For this review, take the finished solid that the model builds, in its own axes (mm). A direction names the side the tool comes from. Give positions to 0.01 mm unless a question says otherwise; leave off trailing zeros. Write each loop counter-clockwise with the first axis right and the second up, starting at its lowest first coordinate (ties: lowest second). Pieces come first, ordered by that corner, then holes. Notation, with made-up numbers: M 5.5,25 L 39.5,25 A22 ccw 39.5,39 Z; hole C 63.5,72.5 d6. An arc over 180 degrees is marked long. One line per item, written item: value. Start each with the question number.
Item 1: Clearance check with flat-ended pins moving along their axes: pin 1 Ø6 at (x, z) = (-14, -16.5) entering from +Y; pin 2 Ø6 at (y, z) = (24, -9) entering from +X; pin 3 Ø8 at (y, z) = (10, -28) entering from +X. State where each tip first meets the part, or that it passes through.
Item 2: Consider section B-B, the plane z = -27.5. Write out the cut boundary in (x, y).
Item 3: Consider section A-A, the plane x = -13. Write out the cut boundary in (y, z), and give its area (3 significant figures).
Item 4: Tool access review of faces 5 (the face through (-36, 27, -20)), 6 (the face through (-38, 40, -20)): name each direction out of +Z, -Z, +X, -X, +Y, -Y from which nothing blocks a thin tool from reaching the whole face with its end or side.
Item 5: Consider section D-D, the plane z = -20.5. Write out the cut boundary in (x, y).
Item 6: Consider section C-C, the plane y = 27. Write out the cut boundary in (x, z).
Item 7: Mouldability with a two-part tool opening along Z and no side actions: class faces 1 (the face through (-37.972, 24.804, -12.012)), 2 (the face through (-32, 8, -40)), 3 (the face through (0, 2, -20)), 4 (the face through (-13.488, 2.028, -25.304)) as released by +Z, released by -Z, zero draft, split by the parting line, or undercut.
Item 8: To check wall thickness, follow probe 1 along Z at (x, y) = (-13, 2.2); probe 2 along Y at (x, z) = (-38.35, -12.5); probe 3 along X at (y, z) = (30, -7). State the ranges of each line that lie inside material, in increasing order.
```python
from build123d import *

# Parameters (mm, degrees)
SCHIZZO1_W                   = 40
SCHIZZO1_H                   = 40
ESTRUSIONE_ESTRUSIONE1_DEPTH = 4
SCHIZZO2_W                   = 4
SCHIZZO2_H                   = 40
ESTRUSIONE_ESTRUSIONE2_DEPTH = 36
SMUSSO1_SIZE                 = 10
FORO_PER_VITE_M4_1_D         = 4.5
FORO_PER_VITE_M4_1_DEPTH     = 9
FORO_PER_VITE_M4_1_TIP       = 1.351936393
FORO_PER_VITE_M4_3_D         = 4.5
FORO_PER_VITE_M4_3_DEPTH     = 9
FORO_PER_VITE_M4_3_TIP       = 1.351936393


with BuildPart() as part:
    # Schizzo1 → Estrusione-Estrusione1 (new body)
    with BuildSketch(Plane(origin=(0, 0, 0), x_dir=(1, 0, 0), z_dir=(0, 1, 0))):
        with Locations((-20, 20)):
            Rectangle(SCHIZZO1_W, SCHIZZO1_H)
    extrude(amount=ESTRUSIONE_ESTRUSIONE1_DEPTH)

    # Schizzo2 → Estrusione-Estrusione2 (add)
    with BuildSketch(Plane(origin=(0, 4, 0), x_dir=(1, 0, 0), z_dir=(0, 1, 0))):
        with Locations((-38, 20)):
            Rectangle(SCHIZZO2_W, SCHIZZO2_H)
    extrude(amount=ESTRUSIONE_ESTRUSIONE2_DEPTH)

    # Smusso1
    smusso1_edges = [part.edges().sort_by_distance(p)[0] for p in [
        (-36, 4, -20),
    ]]
    chamfer(smusso1_edges, length=SMUSSO1_SIZE)

    # Foro per Vite M4-1
    with Locations(Plane(origin=(0, 0, 0), x_dir=(-1, 0, 0), z_dir=(0, -1, 0))):
        with Locations((13, 27.5), (13, 12.5)):
            Hole(FORO_PER_VITE_M4_1_D / 2, depth=FORO_PER_VITE_M4_1_DEPTH)
            with Locations((0, 0, -(FORO_PER_VITE_M4_1_DEPTH + FORO_PER_VITE_M4_1_TIP / 2))):  # 118° drill point
                Cone(0, FORO_PER_VITE_M4_1_D / 2, FORO_PER_VITE_M4_1_TIP, mode=Mode.SUBTRACT)

    # Foro per Vite M4-3
    with Locations(Plane.ZY.offset(40)):
        with Locations((-27.5, 27), (-12.5, 27)):
            Hole(FORO_PER_VITE_M4_3_D / 2, depth=FORO_PER_VITE_M4_3_DEPTH)
            with Locations((0, 0, -(FORO_PER_VITE_M4_3_DEPTH + FORO_PER_VITE_M4_3_TIP / 2))):  # 118° drill point
                Cone(0, FORO_PER_VITE_M4_3_D / 2, FORO_PER_VITE_M4_3_TIP, mode=Mode.SUBTRACT)


solid = part.part
```
Model answer:
1. pin 1: stops at y = 4
1. pin 2: stops at x = -36
1. pin 3: stops at x = -28
2. outline: M -40,0 L -15.25,0 L -15.25,4 L -26,4 L -36,14 L -36,24.75 L -40,24.75 Z; M -40,29.25 L -36,29.25 L -36,40 L -40,40 Z; M -10.75,0 L 0,0 L 0,4 L -10.75,4 Z
3. outline: M 0,-40 L 4,-40 L 4,-29.75 L 0,-29.75 Z; M 0,-25.25 L 4,-25.25 L 4,-14.75 L 0,-14.75 Z; M 0,-10.25 L 4,-10.25 L 4,0 L 0,0 Z
3. area: 124 mm2
4. face 5: +Z, -Z, +X, +Y
4. face 6: +Z, -Z, +X, -X, +Y
5. outline: M -40,0 L 0,0 L 0,4 L -26,4 L -36,14 L -36,40 L -40,40 Z
6. outline: M -40,-40 L -36,-40 L -36,-29.75 L -40,-29.75 Z; M -40,-25.25 L -36,-25.25 L -36,-14.75 L -40,-14.75 Z; M -40,-10.25 L -36,-10.25 L -36,0 L -40,0 Z
7. face 1: undercut
7. face 2: released by -Z
7. face 3: zero draft
7. face 4: undercut
8. probe 1: z = -40 to -29.75, -25.25 to -14.75, -10.25 to 0
8. probe 2: y = 0 to 24.75, 29.25 to 40
8. probe 3: x = -40 to -36
